Model file for the job. Use its own axes, mm. A direction names the side the tool comes from. Round coordinates to 2 decimals unless told otherwise and drop trailing zeros. Loops run counter-clockwise (first coordinate to the right, second up) from the corner with the lowest first, then second, coordinate; pieces in that order, holes last. Notation, with made-up numbers: M 67.5,72.5 L 71.5,72.5 A11 cw 71.5,77.5 Z; hole C -28.75,30 d6. An arc over 180 degrees is marked long. Use a Markdown table: item, result. Add a question column.
Q1. Mould opens along X. For faces 3 (the face through (10, 21, -36)), 4 (the face through (-0.521, 1.268, -18.966)), 5 (the face through (0, 0, -1)), 6 (the face through (-0.867, 51.095, -36.232)) say: +X half, -X half, draft (parallel to the pull), parting line (faces both ways), or undercut.
Q2. Tool access for faces 1 (the face through (0, 2.5, 1)), 2 (the face through (-0.521, 26.466, -36.232)): list every direction of +Z, -Z, +X, -X, +Y, -Y with a clear straight run to the whole face (end or side of a thin tool).
Q3. Probe line 1 (Z direction, x = 0, y = 1.3); line 2 (Y direction, x = 0, z = -35.8); line 3 (Z direction, x = -7.5, y = 13). List the from-to ranges inside material, lowest first. Write a range as from..to.
Q4. Cut at C-C (x = 0). Give the cut face in (y, z).
Q5. Cut at B-B (z = -15). Give the cut face in (x, y), plus the area to 3 significant figures.
Q6. Cut at A-A (y = 22.5). Give the cut face in (x, z).
Q7. Pin check, flat tips, straight feed: pin 1 (7 mm diameter, centred on x = 0, y = 55, fed in from -Z); pin 2 (12 mm diameter, centred on x = -5.5, y = 47, fed in from +Z); pin 3 (6 mm diameter, centred on x = -5, z = -11.5, fed in from +Y). Stop position of each tip, or through.
Q8. Cut at D-D (x = -5). Give the cut face in (y, z).
from build123d import *

# Parameters (mm, degrees)
SKETCH1_W           = 20
SKETCH1_H           = 75
BOSS_EXTRUDE1_DEPTH = 2.5
SKETCH2_W           = 20
SKETCH2_H           = 2.5
BOSS_EXTRUDE2_DEPTH = 72.5
SKETCH3_R           = 4
CUT_EXTRUDE1_DEPTH  = 2.5
SKETCH4_R           = 4
CUT_EXTRUDE2_DEPTH  = 2.5


with BuildPart() as part:
    # Sketch1 → Boss-Extrude1 (new body)
    with BuildSketch(Plane(origin=(0, 0, 0), x_dir=(1, 0, 0), z_dir=(0, 1, 0))):
        Rectangle(SKETCH1_W, SKETCH1_H)
    extrude(amount=BOSS_EXTRUDE1_DEPTH)

    # Sketch2 → Boss-Extrude2 (add)
    with BuildSketch(Plane(origin=(0, 2.5, 0), x_dir=(1, 0, 0), z_dir=(0, 1, 0))):
        with Locations((0, 36.25)):
            Rectangle(SKETCH2_W, SKETCH2_H)
    extrude(amount=BOSS_EXTRUDE2_DEPTH)

    # Sketch3 → Cut-Extrude1 (cut)
    with BuildSketch(Plane(origin=(0, 2.5, 0), x_dir=(1, 0, 0), z_dir=(0, 1, 0))):
        with Locations((0, 15)):
            Circle(SKETCH3_R)
        with Locations((0, -17.5)):
            Circle(SKETCH3_R)
    extrude(amount=-CUT_EXTRUDE1_DEPTH, mode=Mode.SUBTRACT)

    # Sketch4 → Cut-Extrude2 (cut)
    with BuildSketch(Plane.XY.offset(-35)):
        with Locations((0, 55)):
            Circle(SKETCH4_R)
        with Locations((0, 22.5)):
            Circle(SKETCH4_R)
    extrude(amount=-CUT_EXTRUDE2_DEPTH, mode=Mode.SUBTRACT)


solid = part.part
Checked values:
| question | item | result |
|---|---|---|
| 1 | face 3 | +X half |
| 1 | face 4 | undercut |
| 1 | face 5 | draft |
| 1 | face 6 | undercut |
| 2 | face 1 | +Z, +X, -X, +Y |
| 2 | face 2 | +Z, -Z |
| 3 | line 1 | z = -37.5..-19, -11..13.5, 21.5..37.5 |
| 3 | line 2 | y = 0..18.5, 26.5..51, 59..75 |
| 3 | line 3 | z = -37.5..-35 |
| 4 | outline | M 0,-37.5 L 18.5,-37.5 L 18.5,-35 L 2.5,-35 L 2.5,-19 L 0,-19 Z; M 0,-11 L 2.5,-11 L 2.5,13.5 L 0,13.5 Z; M 0,21.5 L 2.5,21.5 L 2.5,37.5 L 0,37.5 Z; M 26.5,-37.5 L 51,-37.5 L 51,-35 L 26.5,-35 Z; M 59,-37.5 L 75,-37.5 L 75,-35 L 59,-35 Z |
| 5 | outline | M -10,0 L -4,0 L -4,2.5 L -10,2.5 Z; M 4,0 L 10,0 L 10,2.5 L 4,2.5 Z |
| 5 | area | 30.0 mm^2 |
| 6 | outline | M -10,-37.5 L -4,-37.5 L -4,-35 L -10,-35 Z; M 4,-37.5 L 10,-37.5 L 10,-35 L 4,-35 Z |
| 7 | pin 1 | passes through |
| 7 | pin 2 | stops at z = -35 |
| 7 | pin 3 | stops at y = 2.5 |
| 8 | outline | M 0,-37.5 L 75,-37.5 L 75,-35 L 2.5,-35 L 2.5,37.5 L 0,37.5 Z |
